Could you check a few things on this drawing? It's one solid part, dimensions in mm from its lowest x, y, z. Round coordinates to 2 decimals unless told otherwise and drop trailing zeros. Write each loop counter-clockwise with the first axis right and the second up, starting at its lowest first coordinate (ties: lowest second). Pieces come first, ordered by that corner, then holes. Notation, with made-up numbers: (19, 9.25) - (41, 9.25) arc R32 cw to (41, 42.25) - close; hole circle Ø1 at (62.25, 28.5). An arc over 180 degrees is marked (long way). Put each result on its own line as item: value.
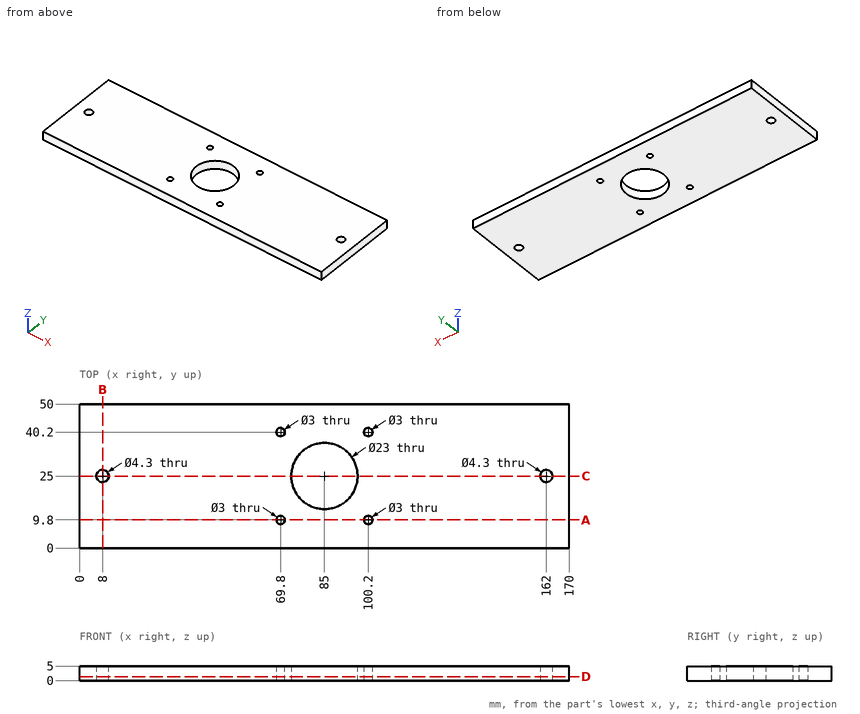
(1) Imagine slicing it at B-B, the plane x = 8. List the corners of the cut face in (y, z) for me, then the cut area to 4 significant figures.
Values found:
outline: (0, 0) - (22.85, 0) - (22.85, 5) - (0, 5) - close; (27.15, 0) - (50, 0) - (50, 5) - (27.15, 5) - close
area: 228.5 mm^2
(2) Imagine slicing it at C-C, the plane y = 25. List the corners of the cut face in (x, z) for me, then the cut area to 3 significant figures.
Values found:
outline: (0, 0) - (5.85, 0) - (5.85, 5) - (0, 5) - close; (10.15, 0) - (73.5, 0) - (73.5, 5) - (10.15, 5) - close; (96.5, 0) - (159.85, 0) - (159.85, 5) - (96.5, 5) - close; (164.15, 0) - (170, 0) - (170, 5) - (164.15, 5) - close
area: 692 mm^2
(3) Please list where these lines run through material, in increasing order: probe 1 along Y at (x, z) = (100.2, 2.7); probe 2 along X at (y, z) = (40.2, 1.6); probe 3 along X at (y, z) = (25, 2.5). Write a range as from..to.
Values found:
probe 1: y = 0..8.3, 11.3..38.7, 41.7..50
probe 2: x = 0..68.3, 71.3..98.7, 101.7..170
probe 3: x = 0..5.85, 10.15..73.5, 96.5..159.85, 164.15..170
(4) Imagine slicing it at A-A, the plane y = 9.8. List the corners of the cut face in (x, z) for me, then the cut area to 3 significant figures.
Values found:
outline: (0, 0) - (68.3, 0) - (68.3, 5) - (0, 5) - close; (71.3, 0) - (98.7, 0) - (98.7, 5) - (71.3, 5) - close; (101.7, 0) - (170, 0) - (170, 5) - (101.7, 5) - close
area: 820 mm^2
(5) Imagine slicing it at D-D, the plane z = 1.3. List the corners of the cut face in (x, y) for me.
Values found:
outline: (0, 0) - (170, 0) - (170, 50) - (0, 50) - close; hole circle Ø4.3 at (8, 25); hole circle Ø3 at (69.8, 9.8); hole circle Ø3 at (69.8, 40.2); hole circle Ø23 at (85, 25); hole circle Ø3 at (100.2, 9.8); hole circle Ø3 at (100.2, 40.2); hole circle Ø4.3 at (162, 25)
